Read the model definition and answer for the solid it produces. Units are mm, in the model's axes. Coordinates: 2 decimals unless noted, no trailing zeros. Order: outer loops, then holes, each group sorted by start corner. A loop starts at its lowest first (then second) coordinate and runs counter-clockwise, first axis right, second up.
```python
from build123d import *

# Parameters (mm, degrees)
SKETCH_1_R      = 3
EXTRUDE_1_DEPTH = 3


with BuildPart() as part:
    # 草图1 → 凸台-拉伸1 (new body)
    with BuildSketch(Plane.XY):
        with BuildLine():
            Line((8.44582472, 166.89164944), (15, 180))
            ThreePointArc((15, 180), (30, 189.270509831), (45, 180))
            Line((45, 180), (51.55417528, 166.89164944))
            ThreePointArc((51.55417528, 166.89164944), (57.859919157, 149.494795444), (60, 131.1145618))
            Line((60, 131.1145618), (60, 125.412430481))
            ThreePointArc((60, 125.412430481), (59.589066182, 121.379009336), (58.373151387, 117.511335106))
            ThreePointArc((58.373151387, 117.511335106), (50.063143822, 62.228284379), (70, 10))
            Line((70, 10), (70, 0))
            Line((70, 0), (60, 0))
            Line((60, 0), (0, 0))
            Line((0, 0), (0, 10))
            Line((0, 10), (0, 131.1145618))
            ThreePointArc((0, 131.1145618), (2.140080843, 149.494795444), (8.44582472, 166.89164944))
        make_face()
        with Locations((10, 10)):
            Circle(SKETCH_1_R, mode=Mode.SUBTRACT)
        with Locations((50, 10)):
            Circle(SKETCH_1_R, mode=Mode.SUBTRACT)
        with Locations((30, 180)):
            Circle(SKETCH_1_R, mode=Mode.SUBTRACT)
    extrude(amount=EXTRUDE_1_DEPTH)


solid = part.part
```
1) Determine the mould class of faces 1 (the cylindrical face through (49.98, 63.02, 1.48)), 2 (the flat face through (11.7, 173.4, 1.5)), 3 (the cylindrical face through (30, 183, 1)), 4 (the flat face through (28, 96, 3)) for opening direction Y: pulls with the +Y half, pulls with the -Y half, needs draft (parallel to the pull), parting line crosses it, or undercut.
A:
face 1: undercut
face 2: pulls with the +Y half
face 3: undercut
face 4: needs draft
2) A cutting plane is placed at A-A, the plane x = 30. Determine the outline of the cut face in (y, z), and give its area (3 significant figures).
A:
outline: (0, 0) - (177, 0) - (177, 3) - (0, 3) - close; (183, 0) - (189.27, 0) - (189.27, 3) - (183, 3) - close
area: 550 mm2
3) Straight lines are drawn through the part: line 1 (X direction, y = 180, z = 1.25); line 2 (Y direction, x = 13.5, z = 0.9); line 3 (X direction, y = 45, z = 1.15). For each, find the intervals that lie inside material, in ascending order.
A:
line 1: x = 15 to 27, 33 to 45
line 2: y = 0 to 177
line 3: x = 0 to 53.33
4) A flat-ended cylindrical pin translates along its axis: pin 1 Ø3.5 at (x, y) = (50, 10) entering from +Z. Find the tip coordinate at first contact, or state that the pin passes through.
A:
pin 1: passes through
5) A cutting plane is placed at B-B, the plane z = 1.25. Determine the outline of the cut face in (x, y), and give its area (3 significant figures).
A:
outline: (0, 0) - (70, 0) - (70, 10) arc R110 cw to (58.37, 117.51) arc R20 ccw to (60, 125.41) - (60, 131.11) arc R80 ccw to (51.55, 166.89) - (45, 180) arc R16.77 ccw to (15, 180) - (8.45, 166.89) arc R80 ccw to (0, 131.11) - close; hole circle Ø6 at (10, 10); hole circle Ø6 at (30, 180); hole circle Ø6 at (50, 10)
area: 9,920 mm2
6) A cutting plane is placed at C-C, the plane y = 135. Determine the outline of the cut face in (x, z), and give its area (3 significant figures).
A:
outline: (0.09, 0) - (59.91, 0) - (59.91, 3) - (0.09, 3) - close
area: 179 mm2
7) A cutting plane is placed at D-D, the plane x = 20.5. Determine the outline of the cut face in (y, z).
A:
outline: (0, 0) - (186.32, 0) - (186.32, 3) - (0, 3) - close
